Input: part model. Units: mm. Frame: model coordinates. A direction names the side the tool comes from. Give positions to 0.01 mm unless a question says otherwise; leave off trailing zeros. Loops run counter-clockwise (first coordinate to the right, second up) from the corner with the lowest first, then second, coordinate; pieces in that order, holes last. Notation, with made-up numbers: (0.25, 33) - (39.25, 33) arc R35 ccw to (39.25, 71) - close; hole circle Ø9 at (0, 75.25). An arc over 180 degrees is marked (long way). One line per item, written item: value.
from build123d import *

# Parameters (mm, degrees)
F1_R          = 11.5
F2_DEPTH      = 19.51505
F2_DEPTH_BACK = 10
F0_R          = 8.875
F3_DEPTH      = 25
F3_DEPTH_BACK = 25
F5_DEPTH      = 25
F5_DEPTH_BACK = 25
F6_W          = 31.0526300933
F6_H          = 13.8705706969
F6_H_2        = 13.1759493425
F7_DEPTH      = 25
F7_DEPTH_BACK = 25
F8_SIZE       = 0.5
F9_R          = 0.5
F10_DEPTH     = 9.3
F11_DEPTH     = 9.7


with BuildPart() as f2:
    # F1 (on Top) → F2 (new body, two sides)
    with BuildSketch(Plane.XY) as f2_sk:
        Circle(F1_R)
    extrude(amount=F2_DEPTH)
    extrude(f2_sk.sketch, amount=-F2_DEPTH_BACK)

    # F0 (on Front) → F3 (cut, two sides)
    with BuildSketch(Plane.XZ) as f3_sk:
        Circle(F0_R)
    extrude(amount=-F3_DEPTH, mode=Mode.SUBTRACT)
    extrude(f3_sk.sketch, amount=F3_DEPTH_BACK, mode=Mode.SUBTRACT)

    # F4 (on Front) → F5 (cut, two sides)
    with BuildSketch(Plane.XZ) as f5_sk:
        Polygon((24.7668549418, 28.5545103252), (-16.3316316903, 28.5545103252), (24.7668549418, -1.7773286672), align=None)
    extrude(amount=-F5_DEPTH, mode=Mode.SUBTRACT)
    extrude(f5_sk.sketch, amount=F5_DEPTH_BACK, mode=Mode.SUBTRACT)

    # F6 (on Top) → F7 (cut, two sides)
    with BuildSketch(Plane.XY) as f7_sk:
        with Locations((1.910218969, 10.3145037405)):
            Rectangle(F6_W, F6_H)
        with Locations((1.910218969, -13.2087562792)):
            Rectangle(F6_W, F6_H_2)
    extrude(amount=-F7_DEPTH, mode=Mode.SUBTRACT)
    extrude(f7_sk.sketch, amount=F7_DEPTH_BACK, mode=Mode.SUBTRACT)

    # F8
    f8_edges = [f2.edges().sort_by_distance(p)[0] for p in [
        (-8.875, 3.379218, 0),
        (-8.875, -6.620782, 0),
    ]]
    chamfer(f8_edges, length=F8_SIZE)

    # F9 (on Top) → F10 (cut)
    with BuildSketch(Plane.XY):
        with BuildLine():
            ThreePointArc((-2.2312842775, 0.1235368601), (-2.7262590243, -0.081488393), (-2.9312842775, -0.5764631399))
            Line((-2.9312842775, -0.5764631399), (-2.9312842775, -2.6688878175))
            ThreePointArc((-2.9312842775, -2.6688878175), (-2.7262590243, -3.1638625643), (-2.2312842775, -3.3688878175))
            ThreePointArc((-2.2312842775, -3.3688878175), (-1.7363095307, -3.1638625643), (-1.5312842775, -2.6688878175))
            Line((-1.5312842775, -2.6688878175), (-1.5312842775, -0.5764631399))
            ThreePointArc((-1.5312842775, -0.5764631399), (-1.7363095307, -0.081488393), (-2.2312842775, 0.1235368601))
        make_face()
        with BuildLine():
            ThreePointArc((0.0221650116, 0.1235368601), (-0.4728097352, -0.081488393), (-0.6778349884, -0.5764631399))
            Line((-0.6778349884, -0.5764631399), (-0.6778349884, -2.6688878175))
            ThreePointArc((-0.6778349884, -2.6688878175), (-0.4728097352, -3.1638625643), (0.0221650116, -3.3688878175))
            ThreePointArc((0.0221650116, -3.3688878175), (0.5171397584, -3.1638625643), (0.7221650116, -2.6688878175))
            Line((0.7221650116, -2.6688878175), (0.7221650116, -0.5764631399))
            ThreePointArc((0.7221650116, -0.5764631399), (0.5171397584, -0.081488393), (0.0221650116, 0.1235368601))
        make_face()
        with Locations((0.0201533299, -1.6274178245)):
            Circle(F9_R, mode=Mode.SUBTRACT)
        with BuildLine():
            ThreePointArc((2.2751650116, 0.1235368601), (1.7801902648, -0.081488393), (1.5751650116, -0.5764631399))
            Line((1.5751650116, -0.5764631399), (1.5751650116, -2.6688878175))
            ThreePointArc((1.5751650116, -2.6688878175), (1.7801902648, -3.1638625643), (2.2751650116, -3.3688878175))
            ThreePointArc((2.2751650116, -3.3688878175), (2.7701397584, -3.1638625643), (2.9751650116, -2.6688878175))
            Line((2.9751650116, -2.6688878175), (2.9751650116, -0.5764631399))
            ThreePointArc((2.9751650116, -0.5764631399), (2.7701397584, -0.081488393), (2.2751650116, 0.1235368601))
        make_face()
    extrude(amount=F10_DEPTH, mode=Mode.SUBTRACT)

    # F9 (on Top) → F11 (cut)
    with BuildSketch(Plane.XY):
        with Locations((0.0201533299, -1.6274178245)):
            Circle(F9_R)
    extrude(amount=F11_DEPTH, mode=Mode.SUBTRACT)


solid = f2.part
Item 1: Draft query along Y for faces 3 (the face through (-2, -2, 9.3)), 4 (the face through (11.346, -1.878, -0.082)), 5 (the face through (-2, -6.621, 12)). Return one class per face: pulls with the +Y half, pulls with the -Y half, needs draft (parallel to the pull), parting line crosses it, or undercut.
Verdict:
face 3: undercut
face 4: parting line crosses it
face 5: pulls with the -Y half
Item 2: Pin query (flat end, axial travel): P1, Ø8, axis at x = -7, z = -3, coming from the +Y side; P2, Ø0.5, axis at y = -2, z = 9, coming from the +X side; P3, Ø1.5, axis at y = 2.5, z = 10, coming from the -X side. Return the tip coordinate at first contact, or that it passes through.
Verdict:
P1: stops at y = 3.38
P2: stops at x = 10.5
P3: stops at x = -11.37
Item 3: Access query for faces 1 (the face through (-8, -2, 19.515)), 2 (the face through (2, -2, 9.3)). Directions: +Z, -Z, +X, -X, +Y, -Y. A direction counts if a zero-diameter tool reaches every point of the face in a straight line with its end or side. Return the directions, or none.
Verdict:
face 1: +Z, +X, -X, +Y, -Y
face 2: none
Item 4: Material intervals for L1, parallel to X at y = -0.75, z = 0 (3 decimals); L2, parallel to X at y = -2.5, z = 2.75; L3, parallel to Z at x = 4.75, y = -2.25, sorted ascending.
Verdict:
L1: x = -11.476 to -8.875, 8.875 to 11.476
L2: x = -11.22 to -8.44, 8.44 to 11.22
L3: z = -10 to -7.5, 7.5 to 13
Item 5: Section C-C, the plane z = 12.25. Output: boundary loops of the cut face in (x, y).
Verdict:
outline: (-10.99, 3.38) arc R11.5 ccw to (-9.4, -6.62) - (5.76, -6.62) - (5.76, 3.38) - close
Item 6: Section A-A, the plane z = 0. Output: boundary loops of the cut face in (x, y) (3 decimals), and give its area (3 significant figures).
Verdict:
outline: (-10.992, 3.379) arc R11.5 ccw to (-9.403, -6.621) - (-9.375, -6.621) - (-8.875, -6.121) - (-8.875, 2.879) - (-9.375, 3.379) - close; (8.875, -6.121) - (9.375, -6.621) - (9.403, -6.621) arc R11.5 ccw to (10.992, 3.379) - (9.375, 3.379) - (8.875, 2.879) - close
area: 42.0 mm^2
